Autodesk Inventor part; units mm, degrees
ref_plane "YZ Plane" through (0, 0, 0) normal (1, 0, 0) x (0, 1, 0)
ref_plane "XZ Plane" through (0, 0, 0) normal (0, 1, 0) x (-1, 0, 0)
ref_plane "XY Plane" through (0, 0, 0) normal (0, 0, 1) x (1, 0, 0)
sketch "Sketch1" plane through (0, 0, 0) normal (0, 0, 1) x (1, 0, 0)
  line L0 (-10, -10) -> (-5.6, -10)
  line L1 (-10, -5.6) -> (-10, -10)
  line L2 (-5.6, -10) -> (-5, -10)
  line L3 (-3.2, -8.2) -> (-5.6, -8.2)
  line L4 (-2.8351, -3.825) -> (-5.6, -6.5899)
  line L5 (-3.825, -2.8351) -> (-6.5899, -5.6)
  line L6 (0, 0) -> (0, -11) construction
  line L7 (0, 0) -> (-12, 0) construction
  line L8 (-3.2, -8.2) -> (-5, -10)
  line L9 (-6.5899, -5.6) -> (-8.2, -5.6)
  line L10 (-10, -5.6) -> (-10, -5)
  line L11 (-10, -5) -> (-8.2, -3.2)
  line L12 (-8.2, -3.2) -> (-8.2, -5.6)
  line L13 (-5.6, -8.2) -> (-5.6, -6.5899)
  arc A0 (-2.15, 0) -> (0, -2.15) centre (0, 0) ccw
  line L14 (0, 0) -> (-3.825, 0)
  line L15 (-3.825, 0) -> (-3.825, -2.8351)
  line L16 (-2.8351, -3.825) -> (0, -3.825)
  line L17 (0, -3.825) -> (0, 0)
  line L18 (-2.8351, -3.825) -> (-3.825, -3.825) construction
  line L19 (-3.825, -3.825) -> (-3.825, -2.8351) construction
  line L20 (3.825, -2.8351) -> (3.825, -3.825) construction
  line L21 (3.825, -2.8351) -> (3.825, 0)
  line L22 (3.825, -3.825) -> (2.8351, -3.825) construction
  line L23 (3.825, 0) -> (0, 0)
  line L24 (0, -3.825) -> (2.8351, -3.825)
  arc A1 (0, -2.15) -> (2.15, 0) centre (0, 0) ccw
  line L25 (0, 0) -> (0, -3.825)
  line L26 (2.8351, -3.825) -> (5.6, -6.5899)
  line L27 (0, 0) -> (0, -12) construction
  line L28 (0, 0) -> (11, 0) construction
  line L29 (3.825, -2.8351) -> (6.5899, -5.6)
  line L30 (8.2, -3.2) -> (8.2, -5.6)
  line L31 (10, -5.6) -> (10, -5)
  line L32 (8.2, -3.2) -> (10, -5)
  line L33 (8.2, -5.6) -> (6.5899, -5.6)
  line L34 (5.6, -6.5899) -> (5.6, -8.2)
  line L35 (10, -10) -> (10, -5.6)
  line L36 (5.6, -10) -> (10, -10)
  line L37 (3.2, -8.2) -> (5.6, -8.2)
  line L38 (5, -10) -> (3.2, -8.2)
  line L39 (5.6, -10) -> (5, -10)
  line L40 (2.8351, 3.825) -> (3.825, 3.825) construction
  line L41 (2.8351, 3.825) -> (0, 3.825)
  line L42 (3.825, 3.825) -> (3.825, 2.8351) construction
  line L43 (0, 3.825) -> (0, 0)
  line L44 (3.825, 0) -> (3.825, 2.8351)
  arc A2 (2.15, 0) -> (0, 2.15) centre (0, 0) ccw
  line L45 (0, 0) -> (3.825, 0)
  line L46 (3.825, 2.8351) -> (6.5899, 5.6)
  line L47 (0, 0) -> (12, 0) construction
  line L48 (0, 0) -> (0, 11) construction
  line L49 (2.8351, 3.825) -> (5.6, 6.5899)
  line L50 (3.2, 8.2) -> (5.6, 8.2)
  line L51 (5.6, 10) -> (5, 10)
  line L52 (3.2, 8.2) -> (5, 10)
  line L53 (5.6, 8.2) -> (5.6, 6.5899)
  line L54 (6.5899, 5.6) -> (8.2, 5.6)
  line L55 (10, 10) -> (5.6, 10)
  line L56 (10, 5.6) -> (10, 10)
  line L57 (8.2, 3.2) -> (8.2, 5.6)
  line L58 (10, 5) -> (8.2, 3.2)
  line L59 (10, 5.6) -> (10, 5)
  line L60 (-3.825, 2.8351) -> (-3.825, 3.825) construction
  line L61 (-3.825, 2.8351) -> (-3.825, 0)
  line L62 (-3.825, 3.825) -> (-2.8351, 3.825) construction
  line L63 (-3.825, 0) -> (0, 0)
  line L64 (0, 3.825) -> (-2.8351, 3.825)
  arc A3 (0, 2.15) -> (-2.15, 0) centre (0, 0) ccw
  line L65 (0, 0) -> (0, 3.825)
  line L66 (-2.8351, 3.825) -> (-5.6, 6.5899)
  line L67 (0, 0) -> (0, 12) construction
  line L68 (0, 0) -> (-11, 0) construction
  line L69 (-3.825, 2.8351) -> (-6.5899, 5.6)
  line L70 (-8.2, 3.2) -> (-8.2, 5.6)
  line L71 (-10, 5.6) -> (-10, 5)
  line L72 (-8.2, 3.2) -> (-10, 5)
  line L73 (-8.2, 5.6) -> (-6.5899, 5.6)
  line L74 (-5.6, 6.5899) -> (-5.6, 8.2)
  line L75 (-10, 10) -> (-10, 5.6)
  line L76 (-5.6, 10) -> (-10, 10)
  line L77 (-3.2, 8.2) -> (-5.6, 8.2)
  line L78 (-5, 10) -> (-3.2, 8.2)
  line L79 (-5.6, 10) -> (-5, 10)
  point P0 (0, 2.15)
  point P1 (2.15, 0)
  point P2 (0, -2.15)
  dimension "d16" = 10
  dimension "d19" = 3.2
  dimension "d21" = 4.4
  dimension "d22" = 4.4
  dimension "d24" = 45
  dimension "d25" = 1.8
  dimension "d27" = 1.8
  dimension "d28" = 45
  dimension "d29" = 3.2
  dimension "d31" = 1.4
  dimension "d33" = 2.15
  dimension "d34" = 3.825
  dimension "d35" = 3.825
  dimension "d36" = 135
  dimension "d39" = 360
extrude "Extrusion1" add sketch "Sketch1" along normal blind 200 contours L1 L10 L11 L12 L9 L5 L15 L14 A0 L17 L16 L4 L13 L3 L8 L2 L0 | L17 A1 L23 L21 L29 L33 L30 L32 L31 L35 L36 L39 L38 L37 L34 L26 L24 | L61 L69 L73 L70 L72 L71 L75 L76 L79 L78 L77 L74 L66 L64 L43 A3 L14 | A2 L43 L41 L49 L53 L50 L52 L51 L55 L56 L59 L58 L57 L54 L46 L44 L23
pattern_linear "Rectangular Pattern1" count 2 spacing 20 along (0, -1, 0) of "Extrusion1"
sketch "Sketch2" plane through (0, 0, 200) normal (0, 0, 1) x (1, 0, 0)
  line L0 (3.2, -8.2) -> (5, -10)
  line L1 (-3.2, -11.8) -> (-5, -10)
  line L2 (5, -10) -> (-5, -10) construction
  line L3 (-8.2, -12.25) -> (8.2, -12.25)
  line L4 (8.2, -12.25) -> (8.2, -7.75)
  line L5 (8.2, -7.75) -> (-8.2, -7.75)
  line L6 (-8.2, -7.75) -> (-8.2, -12.25)
  line L7 (-8.2, -12.25) -> (8.2, -7.75) construction
  line L8 (8.2, -12.25) -> (-8.2, -7.75) construction
  line L9 (10, -15) -> (10, -5)
  line L10 (5.6, -6.5899) -> (5.6, -8.2)
  line L11 (5.6, -6.5899) -> (6.7601, -7.75)
  line L12 (-5.6, -6.5899) -> (-2.8351, -3.825)
  line L13 (-5.6, -6.5899) -> (-6.7601, -7.75)
  line L14 (5.6, -13.4101) -> (6.7601, -12.25)
  line L15 (-5.6, -13.4101) -> (-6.7601, -12.25)
  line L16 (-5.6, -6.5899) -> (-5.6, -7.75)
  line L17 (-5.6, -8.2) -> (-5.6, -6.5899)
  line L18 (5.6, -6.5899) -> (5.6, -7.75)
  line L19 (-5.6, -11.8) -> (-5.6, -13.4101)
  line L20 (5.6, -13.4101) -> (5.6, -12.25)
  point P0 (0, 0)
  point P1 (0, -10)
  point P2 (-5.6, -12.25)
  dimension "d46" = 4.5
  dimension "d50" = 1.8
extrude "Extrusion2" cut sketch "Sketch2" against normal through all
properties part number "AP20x20"
Input: part model. Units: mm. Frame: model coordinates. A direction names the side the tool comes from. Round coordinates to 2 decimals unless told otherwise and drop trailing zeros. Write each loop counter-clockwise with the first axis right and the second up, starting at its lowest first coordinate (ties: lowest second). Pieces come first, ordered by that corner, then holes.
1) Draft query along Y for faces 1 (the flat face through (0, -23.825, 99)), 2 (the flat face through (3.825, -20, 99)), 3 (the flat face through (-10, -27, 99)). Return one class per face: pulls with the +Y half, pulls with the -Y half, needs draft (parallel to the pull), parting line crosses it, or undercut.
2) Cut plane A-A (y = -20). Return the cut outline in (x, z) (3 decimals).
3) Cut plane B-B (x = 0). Return the cut outline in (y, z) (3 decimals).
4) Cut plane C-C (z = 45). Count the separate pieces of the cut face and the enclosed holes in it, then the cut area to 3 significant figures.
5) Reachability of faces 4 (the flat face through (-3.825, -20, 99)), 5 (the flat face through (3.825, 0, 99)), 6 (the flat face through (4.77, -14.24, 98.6)) from +Z, -Z, +X, -X, +Y, -Y: full face, straight path, thin tool, end or side. Return the list, or none.
6) Contact query for flat-ended pins moving along their axis: P1, Ø0.7, axis at y = -4, z = 111.5, coming from the +X side; P2, Ø7, axis at x = 0, y = 0, coming from the +Z side; P3, Ø0.7, axis at x = 4.5, z = 59, coming from the -Y side; P4, Ø4.5, axis at y = 0.5, z = 83.5, coming from the +X side (3 decimals). Output: stop coordinate, or through.
7) Ray query, L1, parallel to Y at x = 0, z = 111 (3 decimals); L2, parallel to Y at x = 7.5, z = 92; L3, parallel to Y at x = -2.75, z = 68 (3 decimals). Return the intervals inside material, ascending.
Geometry says:
1. face 1: pulls with the -Y half
1. face 2: undercut
1. face 3: needs draft
2. outline: (-3.825, 0) - (-2.15, 0) - (-2.15, 200) - (-3.825, 200) - close; (2.15, 0) - (3.825, 0) - (3.825, 200) - (2.15, 200) - close
3. outline: (-23.825, 0) - (-22.15, 0) - (-22.15, 200) - (-23.825, 200) - close; (-17.85, 0) - (-16.175, 0) - (-16.175, 200) - (-17.85, 200) - close; (-3.825, 0) - (-2.15, 0) - (-2.15, 200) - (-3.825, 200) - close; (2.15, 0) - (3.825, 0) - (3.825, 200) - (2.15, 200) - close
4. separate pieces: 1
4. enclosed holes: 3
4. area: 285 mm2
5. face 4: +Z, -Z, -X
5. face 5: +Z, -Z, +X
5. face 6: +Z, -Z
6. P1: stops at x = 9.35
6. P2: stops at z = 200
6. P3: stops at y = -29.85
6. P4: stops at x = 3.825
7. L1: y = -23.825 to -22.15, -17.85 to -16.175, -3.825 to -2.15, 2.15 to 3.825
7. L2: y = -30 to -25.6, -14.4 to -12.25, -7.75 to -5.6, 5.6 to 10
7. L3: y = -23.825 to -16.175, -3.825 to 3.825
